The model under review builds one solid part; all positions refer to its coordinate system, in mm. Face numbers are marked on the shaded views. A direction names the side the tool comes from. Round coordinates to 2 decimals unless told otherwise and drop trailing zeros. Order: outer loops, then holes, each group sorted by start corner. A loop starts at its lowest first (then second) coordinate and runs counter-clockwise, first axis right, second up. Notation, with made-up numbers: M 73,-5.5 L 113,-5.5 A17 cw 113,8.5 Z; hole C -37.5,35.5 d5. An arc over 180 degrees is marked long. Use a Markdown table: item, result. Add a question column.
1. Insertion check: P1, Ø12, axis at y = 10.5, z = 30.5, coming from the -X side; P2, Ø10, axis at x = 45, z = 20, coming from the +Y side; P3, Ø3, axis at x = 3, z = 35, coming from the +Y side. Each pin has a flat end and moves straight along its axis. Give the tip position at first contact, or say it passes through.
2. For the marked faces 1, 2, 3, 4 and 5, list the 3-axis set-ups (+Z, -Z, +X, -X, +Y, -Y) from which the entire face can be reached by the end or side of a thin tool; tool diameter is ignored.
3. Consider section C-C on y = 22. State the section outline as (x, z) points, then the cut area to 3 significant figures.
4. To check wall thickness, follow probe 1 along Z at (x, y) = (27, 16); probe 2 along Y at (x, z) = (40, 5); probe 3 along X at (y, z) = (15, 7). State the ranges of each line that lie inside material, in increasing order.
5. Consider section D-D on z = 47.5. State the section outline as (x, y) points, then the cut area to 3 significant figures.
6. Consider section A-A on z = 25. State the section outline as (x, y) points, then the cut area to 3 significant figures.
7. The part is to be moulded in two halves that separate along Y. For the marked faces 6, 7, 8 and 9, say which applies: +Y half, -Y half, draft (parallel to the pull), parting line (faces both ways), or undercut.
8. Consider section B-B on x = 40. State the section outline as (y, z) points, then the cut area to 3 significant figures.
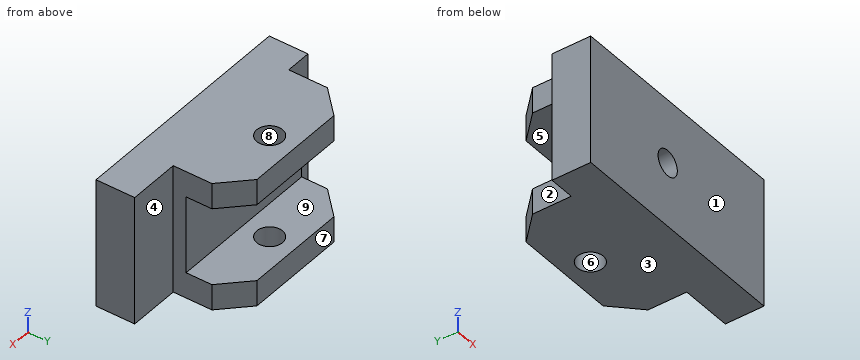
from build123d import *

# Parameters (mm, degrees)
SKETCH3_W                      = 90
SKETCH3_H                      = 15
BOSS_EXTRUDE1_DEPTH            = 50
BOSS_EXTRUDE2_DEPTH            = 50
SKETCH6_W                      = 40
SKETCH6_H                      = 30
CUT_EXTRUDE1_DEPTH             = 20
CUT_EXTRUDE2_REACH             = 91.791
SKETCH7_W                      = 30
SKETCH7_H                      = 14.142135623
CUT_EXTRUDE2_DIRECTION_2_DEPTH = 90.79142498
CUT_EXTRUDE3_DEPTH             = 90.582364336
CUT_EXTRUDE3_DEPTH_BACK        = 90.582364336
SKETCH8_W                      = 30
SKETCH8_H                      = 10
SKETCH9_W                      = 30
SKETCH9_H                      = 14.142135623
CUT_EXTRUDE4_DEPTH             = 10.5
CUT_EXTRUDE5_DEPTH             = 106.948100502
CUT_EXTRUDE5_DEPTH_BACK        = 106.948100502
SKETCH10_R                     = 5
CUT_EXTRUDE6_DEPTH             = 105.880884817
CUT_EXTRUDE6_DEPTH_BACK        = 105.880884817
SKETCH11_R                     = 5


with BuildPart() as part:
    # Sketch3 → Boss-Extrude1 (new body)
    with BuildSketch(Plane.XY):
        with Locations((45, -7.5)):
            Rectangle(SKETCH3_W, SKETCH3_H)
    extrude(amount=BOSS_EXTRUDE1_DEPTH)

    # Sketch5 → Boss-Extrude2 (add)
    with BuildSketch(Plane.XY.offset(50)):
        Polygon((10, 0), (10, 15), (20, 25), (60, 25), (70, 15), (70, 0), align=None)
    extrude(amount=-BOSS_EXTRUDE2_DEPTH)

    # Sketch6 → Cut-Extrude1 (cut)
    with BuildSketch(Plane(origin=(0, 25, 0), x_dir=(1, 0, 0), z_dir=(0, 1, 0))):
        with Locations((40, -25)):
            Rectangle(SKETCH6_W, SKETCH6_H)
    extrude(amount=-CUT_EXTRUDE1_DEPTH, mode=Mode.SUBTRACT)

    # Sketch7 → Cut-Extrude2 (cut, up to next)
    with BuildSketch(Plane(origin=(42.5, 42.5, 0), x_dir=(0, 0, -1), z_dir=(0.7071067811865472, 0.7071067811865479, 0)), mode=Mode.PRIVATE) as cut_extrude2_sk1:
        with Locations((-25, -31.819805153)):
            Rectangle(SKETCH7_W, SKETCH7_H)
    cut_extrude2_tool1 = extrude(cut_extrude2_sk1.sketch, amount=-CUT_EXTRUDE2_REACH, mode=Mode.PRIVATE) & part.part
    add(cut_extrude2_tool1.solids().sort_by_distance((65, 20, 25))[0], mode=Mode.SUBTRACT)

    # Sketch7 → Cut-Extrude2 direction 2 (cut)
    with BuildSketch(Plane(origin=(42.5, 42.5, 0), x_dir=(0, 0, -1), z_dir=(0.7071067811865472, 0.7071067811865479, 0))):
        with Locations((-25, -31.819805153)):
            Rectangle(SKETCH7_W, SKETCH7_H)
    extrude(amount=CUT_EXTRUDE2_DIRECTION_2_DEPTH, mode=Mode.SUBTRACT)

    # Sketch8 → Cut-Extrude3 (cut, two sides: drawn at the far end of the back side and taken through both)
    with BuildSketch(Plane(origin=(70, 0, 0), x_dir=(0, 0, -1), z_dir=(1, 0, 0)).offset(-CUT_EXTRUDE3_DEPTH_BACK)):
        with Locations((-25, 10)):
            Rectangle(SKETCH8_W, SKETCH8_H)
    extrude(amount=CUT_EXTRUDE3_DEPTH + CUT_EXTRUDE3_DEPTH_BACK, mode=Mode.SUBTRACT)

    # Sketch9 → Cut-Extrude4 (cut, symmetric)
    with BuildSketch(Plane(origin=(-2.5, 2.5, 0), x_dir=(0, 0, 1), z_dir=(-0.7071067811865477, 0.7071067811865475, 0))):
        with Locations((25, 24.748737342)):
            Rectangle(SKETCH9_W, SKETCH9_H)
    extrude(amount=CUT_EXTRUDE4_DEPTH, both=True, mode=Mode.SUBTRACT)

    # Sketch10 → Cut-Extrude5 (cut, two sides: drawn at the far end of the back side and taken through both)
    with BuildSketch(Plane.XY.offset(50).offset(-CUT_EXTRUDE5_DEPTH_BACK)):
        with Locations((40, 15)):
            Circle(SKETCH10_R)
    extrude(amount=CUT_EXTRUDE5_DEPTH + CUT_EXTRUDE5_DEPTH_BACK, mode=Mode.SUBTRACT)

    # Sketch11 → Cut-Extrude6 (cut, two sides: drawn at the far end of the back side and taken through both)
    with BuildSketch(Plane(origin=(0, 5, 0), x_dir=(1, 0, 0), z_dir=(0, 1, 0)).offset(-CUT_EXTRUDE6_DEPTH_BACK)):
        with Locations(Location((40, -25, 0), (0, 0, 270))):
            Circle(SKETCH11_R)
    extrude(amount=CUT_EXTRUDE6_DEPTH + CUT_EXTRUDE6_DEPTH_BACK, mode=Mode.SUBTRACT)


solid = part.part
Answer block:
| question | item | result |
|---|---|---|
| 1 | P1 | x = 10 |
| 1 | P2 | y = 5 |
| 1 | P3 | y = 0 |
| 2 | face 1 | +Z, -Z, +X, -X, -Y |
| 2 | face 2 | +Z, -Z, -X, +Y |
| 2 | face 3 | -Z, +X, -X, +Y, -Y |
| 2 | face 4 | +Z, -Z, +X, +Y |
| 2 | face 5 | +X, -X, +Y |
| 3 | outline | M 17,0 L 63,0 L 63,10 L 17,10 Z; M 17,40 L 63,40 L 63,50 L 17,50 Z |
| 3 | area | 920 mm^2 |
| 4 | probe 1 | 0 to 10, 40 to 50 |
| 4 | probe 2 | -15 to 10, 20 to 25 |
| 4 | probe 3 | 10 to 35, 45 to 70 |
| 5 | outline | M 0,-15 L 90,-15 L 90,0 L 70,0 L 70,15 L 60,25 L 20,25 L 10,15 L 10,0 L 0,0 Z; hole C 40,15 d10 |
| 5 | area | 2,670 mm^2 |
| 6 | outline | M 0,-15 L 35,-15 L 35,5 L 10,5 L 10,0 L 0,0 Z; M 45,-15 L 90,-15 L 90,0 L 70,0 L 70,5 L 45,5 Z |
| 6 | area | 1,450 mm^2 |
| 7 | face 6 | undercut |
| 7 | face 7 | +Y half |
| 7 | face 8 | undercut |
| 7 | face 9 | draft |
| 8 | outline | M -15,0 L 10,0 L 10,10 L 5,10 L 5,20 L -15,20 Z; M -15,30 L 5,30 L 5,40 L 10,40 L 10,50 L -15,50 Z; M 20,0 L 25,0 L 25,10 L 20,10 Z; M 20,40 L 25,40 L 25,50 L 20,50 Z |
| 8 | area | 1,000 mm^2 |
